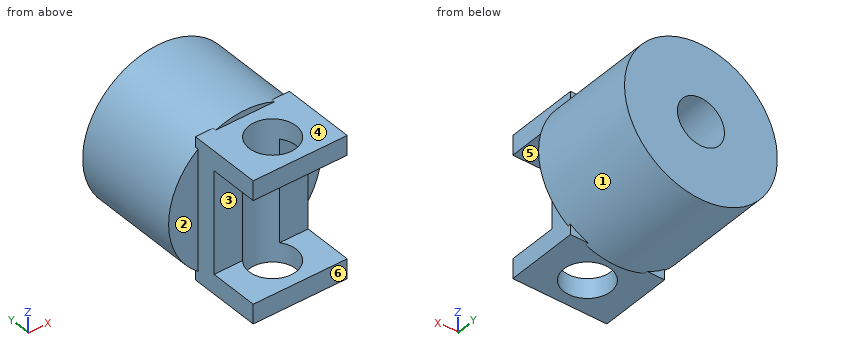
```python
from build123d import *

# Parameters (mm, degrees)
SKETCH1_R           = 32.5
BOSS_EXTRUDE1_DEPTH = 46
SKETCH2_R           = 10
CUT_EXTRUDE1_DEPTH  = 40
BOSS_EXTRUDE2_DEPTH = 20
SKETCH4_R           = 10
CUT_EXTRUDE2_DEPTH  = 42


with BuildPart() as part:
    # Sketch1 → Boss-Extrude1 (new body)
    with BuildSketch(Plane(origin=(0, 0, 0), x_dir=(1, 0, 0), z_dir=(0, 1, 0))):
        Circle(SKETCH1_R)
    extrude(amount=BOSS_EXTRUDE1_DEPTH)

    # Sketch2 → Cut-Extrude1 (cut)
    with BuildSketch(Plane(origin=(0, 46, 0), x_dir=(1, 0, 0), z_dir=(0, 1, 0))):
        Circle(SKETCH2_R)
    extrude(amount=-CUT_EXTRUDE1_DEPTH, mode=Mode.SUBTRACT)

    # Sketch3 → Boss-Extrude2 (add, symmetric)
    with BuildSketch(Plane(origin=(0, 0, 0), x_dir=(0, 0, -1), z_dir=(1, 0, 0))):
        Polygon((30, 1.387692851), (-30, 1.387692851), (-30, -29.525977517), (-21.708955771, -29.525977517), (-21.708955771, -8.612307149), (21.708955771, -8.612307149), (21.708955771, -29.525977517), (30, -29.525977517), align=None)
    extrude(amount=BOSS_EXTRUDE2_DEPTH, both=True)

    # Sketch4 → Cut-Extrude2 (cut, symmetric)
    with BuildSketch(Plane.XY):
        with Locations((0, -14.762988758)):
            Circle(SKETCH4_R)
    extrude(amount=CUT_EXTRUDE2_DEPTH, both=True, mode=Mode.SUBTRACT)


solid = part.part
```
Source: CAD feature listing. Evaluate the final solid. Frame: model axes, mm. Face numbers are marked on the shaded views. A direction names the side the tool comes from. Give positions to 0.01 mm unless a question says otherwise; leave off trailing zeros. Loops run counter-clockwise (first coordinate to the right, second up) from the corner with the lowest first, then second, coordinate; pieces in that order, holes last. Notation, with made-up numbers: (77.25, 51.25) -> (115.25, 51.25) arc R12 ccw to (115.25, 73.25) -> close; hole circle Ø4 at (14, -4). An arc over 180 degrees is marked (long way). Use a Markdown table: item, result. Add a question column.
(1) Pull-direction query (Z, two-part tool) for the marked faces 4, 5 and 6; classes: +Z half, -Z half, draft (parallel to the pull), parting line (faces both ways), or undercut.
(2) Section query B-B (z = -19.5). Output: boundary loops of the cut face in (x, y).
(3) Section query A-A (x = 0). Output: boundary loops of the cut face in (y, z), then the cut area to 3 significant figures.
(4) Ray query, line 1 (Z direction, x = -10.5, y = -16); line 2 (X direction, y = -6.5, z = -7); line 3 (Y direction, x = 0, z = 0). Return the intervals inside material, ascending.
(5) Section query C-C (y = -12). Output: boundary loops of the cut face in (x, z), then the cut area to 3 significant figures.
(6) Access query for the marked faces 1, 2 and 3. Directions: +Z, -Z, +X, -X, +Y, -Y. A direction counts if a zero-diameter tool reaches every point of the face in a straight line with its end or side. Return the directions, or none.
(7) Section query D-D (z = 0). Output: boundary loops of the cut face in (x, y).
(8) First-contact query: pin 1 Ø8 at (x, y) = (-1, 27) entering from -Z; pin 2 Ø4 at (y, z) = (18.5, -23) entering from +X; pin 3 Ø2 at (x, z) = (-0.5, -31.5) entering from -Y. Flat tips, straight axial feed; report the tip coordinate or a pass-through.
Checked values:
| question | item | result |
|---|---|---|
| 1 | face 4 | +Z half |
| 1 | face 5 | undercut |
| 1 | face 6 | draft |
| 2 | outline | (-26, 0) -> (-20, 0) -> (-20, -8.61) -> (-7.88, -8.61) arc R10 cw to (7.88, -8.61) -> (20, -8.61) -> (20, 0) -> (26, 0) -> (26, 46) -> (-26, 46) -> close |
| 3 | outline | (-29.53, -30) -> (-24.76, -30) -> (-24.76, -21.71) -> (-29.53, -21.71) -> close; (-29.53, 21.71) -> (-24.76, 21.71) -> (-24.76, 30) -> (-29.53, 30) -> close; (-4.76, -30) -> (0, -30) -> (0, -32.5) -> (46, -32.5) -> (46, -10) -> (6, -10) -> (6, 10) -> (46, 10) -> (46, 32.5) -> (0, 32.5) -> (0, 30) -> (-4.76, 30) -> close |
| 3 | area | 2,550 mm^2 |
| 4 | line 1 | -30 to -21.71, 21.71 to 30 |
| 4 | line 2 | -20 to -5.63, 5.63 to 20 |
| 4 | line 3 | -4.76 to 6 |
| 5 | outline | (-20, -30) -> (-9.61, -30) -> (-9.61, -21.71) -> (-20, -21.71) -> close; (-20, 21.71) -> (-9.61, 21.71) -> (-9.61, 30) -> (-20, 30) -> close; (9.61, -30) -> (20, -30) -> (20, -21.71) -> (9.61, -21.71) -> close; (9.61, 21.71) -> (20, 21.71) -> (20, 30) -> (9.61, 30) -> close |
| 5 | area | 345 mm^2 |
| 6 | face 1 | +Y |
| 6 | face 2 | +Z, -Z, -X, -Y |
| 6 | face 3 | +X, -X, -Y |
| 7 | outline | (-32.5, 0) -> (-20, 0) -> (-20, -8.61) -> (-7.88, -8.61) arc R10 cw to (7.88, -8.61) -> (20, -8.61) -> (20, 0) -> (32.5, 0) -> (32.5, 46) -> (10, 46) -> (10, 6) -> (-10, 6) -> (-10, 46) -> (-32.5, 46) -> close |
| 8 | pin 1 | z = -32.5 |
| 8 | pin 2 | x = 24.8 |
| 8 | pin 3 | y = 0 |
